from build123d import *

# Parameters (mm, degrees)
BOSS_EXTRU_3_DEPTH      = 6
ENL_V_MAT_EXTRU_1_DEPTH = 10


with BuildPart() as part:
    # Esquisse2 → Boss.-Extru.3 (new body)
    with BuildSketch(Plane(origin=(0, 0, 0), x_dir=(0, 0, -1), z_dir=(1, 0, 0))):
        with BuildLine():
            Line((119.711610695, 366.039005154), (109.711610695, 366.039005154))
            Line((109.711610695, 366.039005154), (109.711610695, 356.039005154))
            Line((109.711610695, 356.039005154), (94.138082152, 356.039005154))
            Line((94.138082152, 356.039005154), (72.155634041, 256.039005154))
            Line((72.155634041, 256.039005154), (54.28830069, 256.039005154))
            Line((54.28830069, 256.039005154), (32.305852578, 156.039005154))
            Line((32.305852578, 156.039005154), (-2.982638809, 156.039005154))
            Line((-2.982638809, 156.039005154), (-38.238065612, 154.511750988))
            Line((-38.238065612, 154.511750988), (-64.527826677, 253.466672484))
            Line((-64.527826677, 253.466672484), (-82.378418708, 252.693390368))
            Line((-82.378418708, 252.693390368), (-108.668179773, 351.648311863))
            Line((-108.668179773, 351.648311863), (-124.227116243, 350.974303556))
            Line((-124.227116243, 350.974303556), (-124.659907248, 360.964933764))
            Line((-124.659907248, 360.964933764), (-134.650537455, 360.532142759))
            add(Edge.make_bspline(
                [(-134.650537455, 360.532142759), (-117.788106266, 213.336232223), (-40.120308472, 162.829698053), (-0.484204579, 40.636249064)],
                knots=[0, 0, 0, 0, 1, 1, 1, 1], degree=3))
            add(Edge.make_bspline(
                [(119.711610695, 366.039005154), (109.23548586, 218.251223276), (33.826338548, 164.430620253), (-0.484204579, 40.636249064)],
                knots=[0, 0, 0, 0, 1, 1, 1, 1], degree=3))
        make_face()
    extrude(amount=BOSS_EXTRU_3_DEPTH)

    # Esquisse3 → Enlèv. mat.-Extru.1 (cut)
    with BuildSketch(Plane(origin=(6, 0, 0), x_dir=(0, 0, -1), z_dir=(1, 0, 0))):
        Polygon((-5.321814798, 54.705223034), (-5.321814798, 81.705223034), (3.678185202, 81.705223034), (3.678185202, 54.705223034), (9.336488724, 34.218680036), (-20.702093174, 34.218680036), align=None)
    extrude(amount=-ENL_V_MAT_EXTRU_1_DEPTH, mode=Mode.SUBTRACT)


solid = part.part
Work out the finished part from the listing and answer in its coordinate system (mm). A direction names the side the tool comes from. Give positions to 0.01 mm unless a question says otherwise; leave off trailing zeros.
Q1. Given pin 1 (1.5 mm diameter, centred on x = 5, z = 5.5, fed in from +Y); pin 2 (2 mm diameter, centred on x = 3.5, y = 177, fed in from +Z); pin 3 (3 mm diameter, centred on x = 4, y = 71.5, fed in from +Z), each flat-ended and moving along its own axis, determine where each tip first touches the part or whether it passes through.
Answer:
pin 1: stops at y = 155.96
pin 2: stops at z = 68.45
pin 3: stops at z = 12.45
Q2. A tool of negligible diameter and unlimited length cuts with its end or side. For faces 3 (the face through (0, 211, 55)), 4 (the face through (2.96, 301.48, 95.34)), from which of +Z, -Z, +X, -X, +Y, -Y can it reach the whole face along a straight path? Write none if from no direction.
Answer:
face 3: +Z, -Z, -X, +Y, -Y
face 4: +X, -X, +Y
Q3. Straight lines are drawn through the part: L1, parallel to Z at x = 4.25, y = 219.5; L2, parallel to Z at x = 2.25, y = 173; L3, parallel to Z at x = 4.75, y = 108.5. For each, find the intervals that lie inside material, in ascending order.
Answer:
L1: z = -80.99 to -46.26, 55.5 to 91.54
L2: z = -57.32 to -36.03, 43.15 to 65.51
L3: z = -24.49 to 28.96
Q4. For a pull along Z with two mould halves and no side action, classify faces 1 (the face through (6, 211, 55)), 2 (the face through (2.96, 206.74, -43.45)) as released by +Z, released by -Z, zero draft, split by the parting line, or undercut.
Answer:
face 1: zero draft
face 2: undercut
